Check sheet for the modelled part. Datum: model origin and axes. Units: mm. Face numbers are marked on the shaded views. A direction names the side the tool comes from. Round coordinates to 2 decimals unless told otherwise and drop trailing zeros. Loops run counter-clockwise (first coordinate to the right, second up) from the corner with the lowest first, then second, coordinate; pieces in that order, holes last. Notation, with made-up numbers: (32.25, -29.5) - (65.25, -29.5) arc R26 ccw to (65.25, -6.5) - close; hole circle Ø5 at (8.25, 40). An arc over 180 degrees is marked (long way). Put each result on its own line as item: value. Start each with the question number.
Item 1: Gauge pin test, flat ends, axial feed: pin 1 Ø14 at (x, y) = (45, -3.5) entering from +Z; pin 2 Ø24 at (x, z) = (-42, 20.5) entering from -Y; pin 3 Ø12 at (y, z) = (-22.5, 2.5) entering from +X. Record the tip position at first contact, or that the pin passes through.
Item 2: Draft check along Y on the marked faces 5, 6 and 7. Enter one of: pulls with the +Y half, pulls with the -Y half, needs draft (parallel to the pull), parting line crosses it, or undercut.
Item 3: Material ranges on line 1 along Z through (x, y) = (-68, 15); line 2 along X through (y, z) = (11.5, 10.5); line 3 along X through (y, z) = (8.5, 7), recorded low to high.
Item 4: Section check D-D, the plane y = -15. Record the cut outline in (x, z), and give its area (3 significant figures).
Item 5: Section check B-B, the plane z = 18. Record the cut outline in (x, y), and give its area (3 significant figures).
Item 6: Section check A-A, the plane x = -63.5. Record the cut outline in (y, z).
Item 7: Tool access check on the marked faces 1, 2, 3 and 4. Record the directions out of +Z, -Z, +X, -X, +Y, -Y that give a thin tool (end or side, any length) a straight path to the whole face; none if there is none.
Item 8: Section check C-C, the plane z = -25.5. Record the cut outline in (x, y).
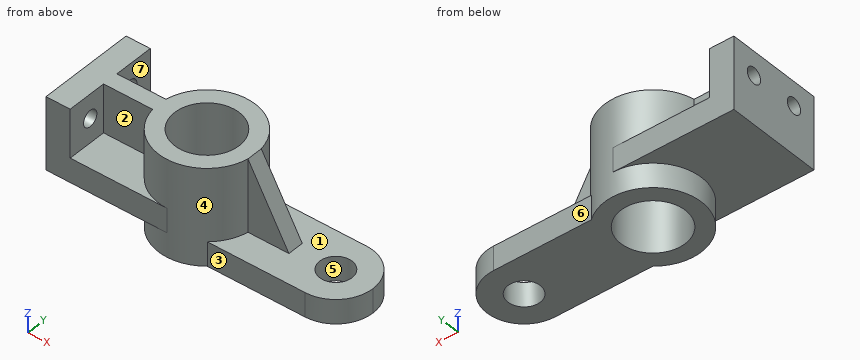
from build123d import *

# Parameters (mm, degrees)
F0_R      = 30
F0_R_2    = 20
F1_DEPTH  = 30
F3_DEPTH  = 15
F4_R      = 10
F5_DEPTH  = 25
F7_DEPTH  = 45
F9_DEPTH  = 35.001
F11_DEPTH = 15
F12_W     = 15
F12_H     = 30
F13_DEPTH = 30
F15_DEPTH = 30
F16_R     = 5
F17_DEPTH = 15.001


with BuildPart() as f1:
    # F0 (on Top) → F1 (new body, symmetric)
    with BuildSketch(Plane.XY):
        Circle(F0_R)
        Circle(F0_R_2, mode=Mode.SUBTRACT)
    extrude(amount=F1_DEPTH, both=True)

    # F2 (on face) → F3 (join)
    with BuildSketch(Plane(origin=(0, 0, -30), x_dir=(1, 0, 0), z_dir=(0, 0, -1))):
        with BuildLine():
            ThreePointArc((103, 0), (96.2634559673, 16.2634559673), (80, 23))
            Line((80, 23), (80, -23))
            ThreePointArc((80, -23), (96.2634559673, -16.2634559673), (103, 0))
        make_face()
        with BuildLine():
            ThreePointArc((80, -23), (57, 0), (80, 23))
            Line((80, 23), (19.2613602843, 23))
            ThreePointArc((19.2613602843, 23), (30, 0), (19.2613602843, -23))
            Line((19.2613602843, -23), (80, -23))
        make_face()
        with BuildLine():
            Line((80, -23), (80, 23))
            ThreePointArc((80, 23), (57, 0), (80, -23))
        make_face()
    extrude(amount=-F3_DEPTH)

    # F4 (on face) → F5 (cut)
    with BuildSketch(Plane.XY.offset(-15)):
        with Locations((80, 0)):
            Circle(F4_R)
    extrude(amount=-F5_DEPTH, mode=Mode.SUBTRACT)

    # F6 (on face) → F7 (join)
    with BuildSketch(Plane.XY.offset(-15)):
        with BuildLine():
            Line((55, 5), (29.5803989155, 5))
            ThreePointArc((29.5803989155, 5), (30, 0), (29.5803989155, -5))
            Line((29.5803989155, -5), (55, -5))
            Line((55, -5), (55, 5))
        make_face()
    extrude(amount=F7_DEPTH)

    # F8 (on face) → F9 (cut, through all)
    with BuildSketch(Plane.XZ.offset(5)):
        Polygon((29.5803989155, 30), (55, -15), (55, 30), align=None)
    extrude(amount=-F9_DEPTH, mode=Mode.SUBTRACT)

    # F10 (on Top) → F11 (join)
    with BuildSketch(Plane.XY):
        with BuildLine():
            ThreePointArc((0, -30), (-30, 0), (0, 30))
            Line((0, 30), (-75, 30))
            Line((-75, 30), (-75, -30))
            Line((-75, -30), (0, -30))
        make_face()
    extrude(amount=-F11_DEPTH)

    # F12 (on Front) → F13 (join, symmetric)
    with BuildSketch(Plane.XZ):
        with Locations((-67.5, 15)):
            Rectangle(F12_W, F12_H)
    extrude(amount=F13_DEPTH, both=True)

    # F14 (on Top) → F15 (join)
    with BuildSketch(Plane.XY):
        with BuildLine():
            Line((-29.5803989155, 5), (-60, 5))
            Line((-60, 5), (-60, -5))
            Line((-60, -5), (-29.5803989155, -5))
            ThreePointArc((-29.5803989155, -5), (-30, 0), (-29.5803989155, 5))
        make_face()
    extrude(amount=F15_DEPTH)

    # F16 (on face) → F17 (cut, through all)
    with BuildSketch(Plane.YZ.offset(-60)):
        with Locations((-15, 15)):
            Circle(F16_R)
        with Locations((15, 15)):
            Circle(F16_R)
    extrude(amount=-F17_DEPTH, mode=Mode.SUBTRACT)


solid = f1.part
Check result:
1. pin 1: z = 15.09
1. pin 2: y = -5
1. pin 3: x = 25.05
2. face 5: undercut
2. face 6: pulls with the +Y half
2. face 7: needs draft
3. line 1: -15 to 10, 20 to 30
3. line 2: -75 to -60, -27.71 to -16.36, 16.36 to 27.71
3. line 3: -75 to -60, -28.77 to -18.1, 18.1 to 28.77
4. outline: (-75, -15) - (-25.98, -15) - (-25.98, -30) - (-13.23, -30) - (-13.23, 30) - (-25.98, 30) - (-25.98, 0) - (-60, 0) - (-60, 10) - (-75, 10) - close; (-75, 20) - (-60, 20) - (-60, 30) - (-75, 30) - close; (13.23, -30) - (97.44, -30) - (97.44, -15) - (25.98, -15) - (25.98, 30) - (13.23, 30) - close
4. area: 3,640 mm²
5. outline: (-75, -30) - (-60, -30) - (-60, -19) - (-75, -19) - close; (-75, -11) - (-60, -11) - (-60, -5) - (-29.58, -5) arc R30 ccw to (29.58, -5) - (36.36, -5) - (36.36, 5) - (29.58, 5) arc R30 ccw to (-29.58, 5) - (-60, 5) - (-60, 11) - (-75, 11) - close; (-75, 19) - (-60, 19) - (-60, 30) - (-75, 30) - close; hole circle Ø40 at (0, 0)
5. area: 2,600 mm²
6. outline: (-30, -15) - (30, -15) - (30, 30) - (-30, 30) - close; hole circle Ø10 at (-15, 15); hole circle Ø10 at (15, 15)
7. face 1: +Z, +X
7. face 2: +Z, -Y
7. face 3: +Z, -Z, +X, -Y
7. face 4: none
8. outline: (19.26, -23) - (80, -23) arc R23 ccw to (80, 23) - (19.26, 23) arc R30 ccw (long way) to start; hole circle Ø40 at (0, 0); hole circle Ø20 at (80, 0)
